from build123d import *

# Parameters (mm, degrees)
SKETCH_R     = 2
PAD_DEPTH    = 3
SKETCH001_W  = 42
SKETCH001_H  = 6.104755
PAD001_DEPTH = 40


with BuildPart() as part:
    # Sketch → Pad (new body)
    with BuildSketch(Plane.XY):
        Polygon((0, 0), (60, 0), (60, 56), (18, 56), (18, 15), (0, 15), align=None)
        with Locations((24.26, 5.6)):
            Circle(SKETCH_R, mode=Mode.SUBTRACT)
        with Locations((41, 5.6)):
            Circle(SKETCH_R, mode=Mode.SUBTRACT)
        with Locations((7.52, 5.6)):
            Circle(SKETCH_R, mode=Mode.SUBTRACT)
    extrude(amount=PAD_DEPTH)

    # Sketch001 → Pad001 (new body)
    with BuildSketch(Plane.XY.offset(3)):
        with Locations((39, 43.052377)):
            Rectangle(SKETCH001_W, SKETCH001_H)
    extrude(amount=PAD001_DEPTH)


solid = part.part
Model file for the job. Use its own axes, mm. A direction names the side the tool comes from. Give positions to 0.01 mm unless a question says otherwise; leave off trailing zeros. Write each loop counter-clockwise with the first axis right and the second up, starting at its lowest first coordinate (ties: lowest second). Pieces come first, ordered by that corner, then holes. Notation, with made-up numbers: (-6.75, 11.5) - (6.25, 11.5) arc R24 cw to (6.25, 23.5) - close; hole circle Ø11 at (60, 60). An arc over 180 degrees is marked (long way). Answer as CSV lines item,"result".
1. 3-axis set-ups, long thin cutter, end or side, ignore diameter. For faces 5 (the face through (39, 51, 3)), 6 (the face through (0, 8, 1)), 7 (the face through (36, 20, 3)): which of +Z, -Z, +X, -X, +Y, -Y reach the whole face in a straight line?
Responses:
face 5,"+Z, +X, -X, +Y"
face 6,"+Z, -Z, -X, +Y, -Y"
face 7,"+Z, +X, -X, -Y"
2. Band-saw the part on B-B (y = 5.6). Write the cut outline in (x, z).
Responses:
outline,"(0, 0) - (5.52, 0) - (5.52, 3) - (0, 3) - close; (9.52, 0) - (22.26, 0) - (22.26, 3) - (9.52, 3) - close; (26.26, 0) - (39, 0) - (39, 3) - (26.26, 3) - close; (43, 0) - (60, 0) - (60, 3) - (43, 3) - close"
3. Band-saw the part on C-C (x = 30). Write the cut outline in (y, z), and give its area (3 significant figures).
Responses:
outline,"(0, 0) - (56, 0) - (56, 3) - (46.1, 3) - (46.1, 43) - (40, 43) - (40, 3) - (0, 3) - close"
area,"412 mm2"
4. Band-saw the part on D-D (z = 31.5). Write the cut outline in (x, y).
Responses:
outline,"(18, 40) - (60, 40) - (60, 46.1) - (18, 46.1) - close"
5. Two-plate mould, pull along X, no slides. Class faces 1 (the face through (60, 40.3, 13.4)), 2 (the face through (18, 40.2, 16.6)), 3 (the face through (42.847, 4.834, 1.479)), 4 (the face through (9, 15, 1)): +X half, -X half, draft (parallel to the pull), parting line (faces both ways), or undercut.
Responses:
face 1,"+X half"
face 2,"-X half"
face 3,"undercut"
face 4,"draft"
6. Pin check, flat tips, straight feed: pin 1 (12 mm diameter, centred on x = 38, z = 19, fed in from -Y); pin 2 (3 mm diameter, centred on x = 46.5, y = 49.5, fed in from +Z); pin 3 (2 mm diameter, centred on x = 51, z = 9.5, fed in from +Y). Stop position of each tip, or through.
Responses:
pin 1,"stops at y = 40"
pin 2,"stops at z = 3"
pin 3,"stops at y = 46.1"
7. Drill centre lines: L1, parallel to Y at x = 24, z = 1; L2, parallel to Z at x = 49, y = 48; L3, parallel to Y at x = 54, z = 20. Where is each one in solid material? Low to high. Write a range as [from, to].
Responses:
L1,"y = [0, 3.62], [7.58, 56]"
L2,"z = [0, 3]"
L3,"y = [40, 46.1]"
8. Band-saw the part on A-A (x = 7.52). Write the cut outline in (y, z).
Responses:
outline,"(0, 0) - (3.6, 0) - (3.6, 3) - (0, 3) - close; (7.6, 0) - (15, 0) - (15, 3) - (7.6, 3) - close"
